The model under review builds one solid part; all positions refer to its coordinate system, in mm. Face numbers are marked on the shaded views. Round coordinates to 2 decimals unless told otherwise and drop trailing zeros. Order: outer loops, then holes, each group sorted by start corner. A loop starts at its lowest first (then second) coordinate and runs counter-clockwise, first axis right, second up. Notation, with made-up numbers: M 19,-0.75 L 32,-0.75 A17 ccw 32,13.25 Z; hole C -31.5,34 d2. An arc over 180 degrees is marked long. Answer as CSV lines item,"result". Start each with the question number.
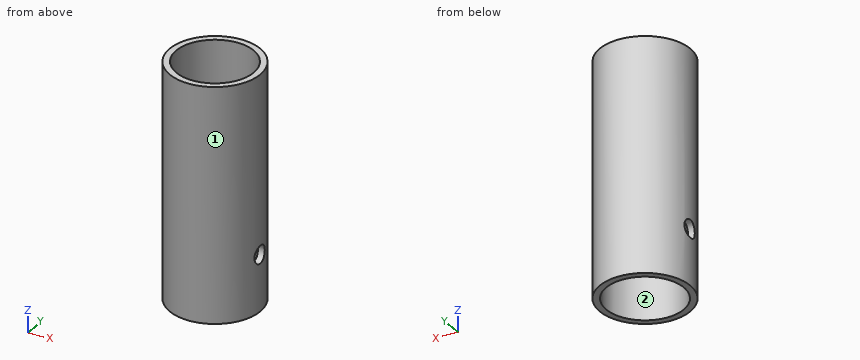
from build123d import *

# Parameters (mm, degrees)
SKETCH1_R               = 4.85
BOSS_EXTRUDE1_DEPTH     = 25
SKETCH2_R               = 4.15
CUT_EXTRUDE1_DEPTH      = 26
SKETCH3_R               = 0.95
CUT_EXTRUDE2_DEPTH      = 5.85
CUT_EXTRUDE2_DEPTH_BACK = 5.85


with BuildPart() as part:
    # Sketch1 → Boss-Extrude1 (new body)
    with BuildSketch(Plane.XY):
        Circle(SKETCH1_R)
    extrude(amount=BOSS_EXTRUDE1_DEPTH)

    # Sketch2 → Cut-Extrude1 (cut, through all)
    with BuildSketch(Plane.XY.offset(25)):
        Circle(SKETCH2_R)
    extrude(amount=-CUT_EXTRUDE1_DEPTH, mode=Mode.SUBTRACT)

    # Sketch3 → Cut-Extrude2 (cut, two sides)
    with BuildSketch(Plane(origin=(0, 0, 0), x_dir=(0, 0, -1), z_dir=(1, 0, 0))) as cut_extrude2_sk:
        with Locations((-6, 0)):
            Circle(SKETCH3_R)
    extrude(amount=CUT_EXTRUDE2_DEPTH, mode=Mode.SUBTRACT)
    extrude(cut_extrude2_sk.sketch, amount=-CUT_EXTRUDE2_DEPTH_BACK, mode=Mode.SUBTRACT)


solid = part.part
Item 1: Consider section B-B (x = 0). State the section outline as (y, z) points.
Item 2: Consider section C-C (z = 6). State the section outline as (x, y) points, and give its area (3 significant figures).
Item 3: Wall thickness on probe 1 along Z at (x, y) = (4.45, 0); probe 2 along Y at (x, z) = (0, 11.25); probe 3 along Y at (x, z) = (3, 14.5): over which ranges is each line inside the solid? List them lowest first. Write a range as [from, to].
Item 4: The part is to be moulded in two halves that separate along X. For the marked faces 1 and 2, say which applies: +X half, -X half, draft (parallel to the pull), parting line (faces both ways), or undercut.
Item 5: For pin 1 (1.5 mm diameter, centred on x = 0, y = 3, fed in from -Z); pin 2 (3 mm diameter, centred on x = -3, z = 8, fed in from -Y), all flat-tipped, find the tip position at first contact; note any pin that passes through.
Item 6: Consider section A-A (y = 0). State the section outline as (x, z) points.
Item 7: Consider section D-D (z = 14.5). State the section outline as (x, y) points.
Reported:
1,outline,"M -4.85,0 L -4.15,0 L -4.15,25 L -4.85,25 Z; M 4.15,0 L 4.85,0 L 4.85,25 L 4.15,25 Z"
2,outline,"M -4.76,-0.95 A4.85 ccw 4.76,-0.95 L 4.04,-0.95 A4.15 cw -4.04,-0.95 Z; M -4.76,0.95 L -4.04,0.95 A4.15 cw 4.04,0.95 L 4.76,0.95 A4.85 ccw Z"
2,area,"17.1 mm²"
3,probe 1,"z = [0, 5.05], [6.95, 25]"
3,probe 2,"y = [-4.85, -4.15], [4.15, 4.85]"
3,probe 3,"y = [-3.81, -2.87], [2.87, 3.81]"
4,face 1,"parting line"
4,face 2,"undercut"
5,pin 1,"passes through"
5,pin 2,"stops at y = -4.61"
6,outline,"M -4.85,0 L -4.15,0 L -4.15,5.05 L -4.85,5.05 Z; M -4.85,6.95 L -4.15,6.95 L -4.15,25 L -4.85,25 Z; M 4.15,0 L 4.85,0 L 4.85,5.05 L 4.15,5.05 Z; M 4.15,6.95 L 4.85,6.95 L 4.85,25 L 4.15,25 Z"
7,outline,"C 0,0 d9.7; hole C 0,0 d8.3"
